from build123d import *

# Parameters (mm, degrees)
PAD015_DEPTH = 12
PAD014_DEPTH = 5


with BuildPart() as body013:
    # Sketch146 → Pad015 (new body)
    with BuildSketch(Plane.XY):
        with BuildLine():
            Line((41.956765, 0.26313), (41.959666, 5.256243))
            ThreePointArc((41.956765, 0.26313), (47.080742, 2.75671), (41.959666, 5.256243))
        make_face()
    extrude(amount=PAD015_DEPTH)


with BuildPart() as body013_1:
    # Body013 placement: moved
    add(body013.part.moved(Location((0, 0, 4))))


with BuildPart() as old_pinion:
    # Sketch145 → Pad014 (new body)
    with BuildSketch(Plane.XY):
        with BuildLine():
            Line((48.939875, 3.670275), (49.473913, 3.767638))
            Line((49.473913, 3.767638), (49.815259, 3.926647))
            Line((49.815259, 3.926647), (50.638101, 4.698494))
            ThreePointArc((50.638101, 4.698494), (50.5458, 4.994259), (50.440501, 5.285649))
            Line((50.440501, 5.285649), (49.318425, 5.40296))
            Line((49.318425, 5.40296), (48.950396, 5.323237))
            Line((48.950396, 5.323237), (48.466153, 5.077911))
            ThreePointArc((47.975725, 5.217399), (48.193585, 5.05148), (48.466153, 5.077911))
            ThreePointArc((47.975725, 5.217399), (47.866498, 5.389716), (47.749972, 5.557185))
            ThreePointArc((47.811432, 6.063346), (47.681442, 5.822318), (47.749972, 5.557185))
            Line((47.811432, 6.063346), (48.225241, 6.414684))
            Line((48.225241, 6.414684), (48.441351, 6.723062))
            Line((48.441351, 6.723062), (48.768029, 7.802923))
            ThreePointArc((48.768029, 7.802923), (48.540212, 8.012912), (48.303325, 8.212614))
            Line((48.303325, 8.212614), (47.272923, 7.75317))
            Line((47.272923, 7.75317), (46.994062, 7.500114))
            Line((46.994062, 7.500114), (46.697359, 7.045533))
            ThreePointArc((46.202892, 6.92112), (46.474523, 6.886359), (46.697359, 7.045533))
            ThreePointArc((46.202892, 6.92112), (46.022139, 7.015737), (45.837491, 7.102506))
            ThreePointArc((45.637635, 7.571584), (45.645575, 7.297853), (45.837491, 7.102506))
            Line((45.637635, 7.571584), (45.820336, 8.082756))
            Line((45.820336, 8.082756), (45.853303, 8.457875))
            Line((45.853303, 8.457875), (45.596285, 9.556401))
            ThreePointArc((45.596285, 9.556401), (45.293995, 9.624348), (44.988994, 9.678852))
            Line((44.988994, 9.678852), (44.326362, 8.765761))
            Line((44.326362, 8.765761), (44.211389, 8.407177))
            Line((44.211389, 8.407177), (44.181727, 7.865147))
            ThreePointArc((43.815712, 7.510168), (44.068332, 7.615881), (44.181727, 7.865147))
            ThreePointArc((43.815712, 7.510168), (43.611867, 7.501733), (43.408573, 7.484553))
            ThreePointArc((43.000954, 7.790859), (43.144695, 7.55777), (43.408573, 7.484553))
            Line((43.000954, 7.790859), (42.903591, 8.324897))
            Line((42.903591, 8.324897), (42.744582, 8.666243))
            Line((42.744582, 8.666243), (41.972735, 9.489085))
            ThreePointArc((41.972735, 9.489085), (41.67697, 9.396784), (41.38558, 9.291486))
            Line((41.38558, 9.291486), (41.268269, 8.169409))
            Line((41.268269, 8.169409), (41.347991, 7.80138))
            Line((41.347991, 7.80138), (41.593318, 7.317138))
            ThreePointArc((41.45383, 6.82671), (41.619749, 7.044569), (41.593318, 7.317138))
            ThreePointArc((41.45383, 6.82671), (41.281512, 6.717482), (41.114044, 6.600956))
            ThreePointArc((40.607883, 6.662416), (40.848911, 6.532426), (41.114044, 6.600956))
            Line((40.607883, 6.662416), (40.256545, 7.076225))
            Line((40.256545, 7.076225), (39.948167, 7.292335))
            Line((39.948167, 7.292335), (38.868306, 7.619013))
            ThreePointArc((38.868306, 7.619013), (38.658317, 7.391196), (38.458615, 7.154309))
            Line((38.458615, 7.154309), (38.918059, 6.123907))
            Line((38.918059, 6.123907), (39.171115, 5.845046))
            Line((39.171115, 5.845046), (39.625696, 5.548343))
            ThreePointArc((39.750109, 5.053876), (39.784869, 5.325508), (39.625696, 5.548343))
            ThreePointArc((39.750109, 5.053876), (39.655491, 4.873124), (39.568723, 4.688475))
            ThreePointArc((39.099644, 4.48862), (39.373376, 4.496559), (39.568723, 4.688475))
            Line((39.099644, 4.48862), (38.588472, 4.67132))
            Line((38.588472, 4.67132), (38.213354, 4.704288))
            Line((38.213354, 4.704288), (37.114828, 4.447269))
            ThreePointArc((37.114828, 4.447269), (37.046881, 4.144979), (36.992377, 3.839978))
            Line((36.992377, 3.839978), (37.905468, 3.177346))
            Line((37.905468, 3.177346), (38.264052, 3.062373))
            Line((38.264052, 3.062373), (38.806082, 3.032711))
            ThreePointArc((39.161061, 2.666696), (39.055348, 2.919317), (38.806082, 3.032711))
            ThreePointArc((39.161061, 2.666696), (39.169495, 2.462852), (39.186676, 2.259557))
            ThreePointArc((38.88037, 1.851938), (39.113458, 1.99568), (39.186676, 2.259557))
            Line((38.88037, 1.851938), (38.346331, 1.754575))
            Line((38.346331, 1.754575), (38.004985, 1.595567))
            Line((38.004985, 1.595567), (37.182144, 0.823719))
            ThreePointArc((37.182144, 0.823719), (37.274445, 0.527954), (37.379743, 0.236564))
            Line((37.379743, 0.236564), (38.50182, 0.119253))
            Line((38.50182, 0.119253), (38.869848, 0.198976))
            Line((38.869848, 0.198976), (39.354091, 0.444302))
            ThreePointArc((39.844519, 0.304814), (39.626659, 0.470733), (39.354091, 0.444302))
            ThreePointArc((39.844519, 0.304814), (39.953746, 0.132497), (40.070272, -0.034972))
            ThreePointArc((40.008813, -0.541133), (40.138803, -0.300105), (40.070272, -0.034972))
            Line((40.008813, -0.541133), (39.595004, -0.892471))
            Line((39.595004, -0.892471), (39.378894, -1.200849))
            Line((39.378894, -1.200849), (39.052216, -2.28071))
            ThreePointArc((39.052216, -2.28071), (39.280033, -2.490699), (39.516919, -2.690401))
            Line((39.516919, -2.690401), (40.547321, -2.230957))
            Line((40.547321, -2.230957), (40.826183, -1.977901))
            Line((40.826183, -1.977901), (41.122886, -1.52332))
            ThreePointArc((41.617353, -1.398907), (41.345721, -1.364146), (41.122886, -1.52332))
            ThreePointArc((41.617353, -1.398907), (41.798105, -1.493524), (41.982754, -1.580293))
            ThreePointArc((42.182609, -2.049371), (42.17467, -1.77564), (41.982754, -1.580293))
            Line((42.182609, -2.049371), (41.999908, -2.560543))
            Line((41.999908, -2.560543), (41.966941, -2.935662))
            Line((41.966941, -2.935662), (42.22396, -4.034188))
            ThreePointArc((42.22396, -4.034188), (42.52625, -4.102135), (42.831251, -4.156639))
            Line((42.831251, -4.156639), (43.493883, -3.243547))
            Line((43.493883, -3.243547), (43.608856, -2.884964))
            Line((43.608856, -2.884964), (43.638518, -2.342934))
            ThreePointArc((44.004532, -1.987955), (43.751912, -2.093668), (43.638518, -2.342934))
            ThreePointArc((44.004532, -1.987955), (44.208377, -1.97952), (44.411672, -1.96234))
            ThreePointArc((44.819291, -2.268646), (44.675549, -2.035557), (44.411672, -1.96234))
            Line((44.819291, -2.268646), (44.916653, -2.802684))
            Line((44.916653, -2.802684), (45.075662, -3.14403))
            Line((45.075662, -3.14403), (45.84751, -3.966872))
            ThreePointArc((45.84751, -3.966872), (46.143275, -3.874571), (46.434665, -3.769273))
            Line((46.434665, -3.769273), (46.551975, -2.647196))
            Line((46.551975, -2.647196), (46.472253, -2.279167))
            Line((46.472253, -2.279167), (46.226926, -1.794925))
            ThreePointArc((46.366415, -1.304496), (46.200495, -1.522356), (46.226926, -1.794925))
            ThreePointArc((46.366415, -1.304496), (46.538732, -1.195269), (46.7062, -1.078743))
            ThreePointArc((47.212362, -1.140203), (46.971333, -1.010213), (46.7062, -1.078743))
            Line((47.212362, -1.140203), (47.563699, -1.554012))
            Line((47.563699, -1.554012), (47.872078, -1.770122))
            Line((47.872078, -1.770122), (48.951939, -2.0968))
            ThreePointArc((48.951939, -2.0968), (49.161928, -1.868983), (49.36163, -1.632096))
            Line((49.36163, -1.632096), (48.902185, -0.601694))
            Line((48.902185, -0.601694), (48.649129, -0.322833))
            Line((48.649129, -0.322833), (48.194549, -0.02613))
            ThreePointArc((48.070135, 0.468337), (48.035375, 0.196706), (48.194549, -0.02613))
            ThreePointArc((48.070135, 0.468337), (48.164753, 0.649089), (48.251522, 0.833738))
            ThreePointArc((48.7206, 1.033593), (48.446869, 1.025654), (48.251522, 0.833738))
            Line((48.7206, 1.033593), (49.231772, 0.850893))
            Line((49.231772, 0.850893), (49.606891, 0.817925))
            Line((49.606891, 0.817925), (50.705417, 1.074944))
            ThreePointArc((50.705417, 1.074944), (50.773364, 1.377234), (50.827868, 1.682235))
            Line((50.827868, 1.682235), (49.914776, 2.344867))
            Line((49.914776, 2.344867), (49.556193, 2.45984))
            Line((49.556193, 2.45984), (49.014163, 2.489502))
            ThreePointArc((48.659184, 2.855517), (48.764896, 2.602897), (49.014163, 2.489502))
            ThreePointArc((48.659184, 2.855517), (48.650749, 3.059361), (48.633569, 3.262656))
            ThreePointArc((48.939875, 3.670275), (48.706786, 3.526534), (48.633569, 3.262656))
        make_face()
    extrude(amount=PAD014_DEPTH)


with BuildPart() as old_pinion_1:
    # Body012 placement: moved
    add(old_pinion.part.moved(Location((0, 0, 4))))

    # Cut001: cut Body013
    add(body013_1.part, mode=Mode.SUBTRACT)


with BuildPart() as old_pinion_2:
    # Cut001 placement: moved
    add(old_pinion_1.part.moved(Location((0, 0, 25.5))))


solid = old_pinion_2.part
Read the model definition and answer for the solid it produces. Units are mm, in the model's axes. A direction names the side the tool comes from. Round coordinates to 2 decimals unless told otherwise and drop trailing zeros. Use one line per item in the form item = value. Start each with the question number.
(1) Flat-ended cylindrical pins translate along their axes: pin 1 Ø1.5 at (x, z) = (39, 30.5) entering from -Y; pin 2 Ø8 at (x, y) = (46.5, 3.5) entering from -Z; pin 3 Ø1 at (y, z) = (7, 33.5) entering from +X; pin 4 Ø1 at (y, z) = (8, 33.5) entering from +X. Find the tip coordinate at first contact, or state that the pin passes through.
(2) For faces 1 (the face through (44.662, 9.229, 31.965)), 2 (the face through (43.158, -3.706, 31.965)), 3 (the face through (38.685, 6.646, 31.965)), determine the directions among +Z, -Z, +X, -X, +Y, -Y from which every point of the face is accessible in a straight line to the end or side of a thin tool.
(3) Determine the mould class of faces 4 (the face through (37.93, 0.18, 31.96)), 5 (the face through (48.602, 7.255, 31.965)), 6 (the face through (49.887, 5.343, 31.965)) for opening direction Y: +Y half, -Y half, draft (parallel to the pull), parting line (faces both ways), or undercut.
(4) Find the intervals of material crossed by line 1 along Y through (x, z) = (38.75, 31.1); line 2 along Y through (x, z) = (50, 30.7); line 3 along Y through (x, z) = (47.75, 33.7), in increasing order. Write a range as from..to.
Checked values:
q1.pin_1 = -2.69
q1.pin_2 = 29.5
q1.pin_3 = 48.68
q1.pin_4 = 48.77
q2.face_1 = +Z, -Z, +Y
q2.face_2 = +Z, -Z, -Y
q2.face_3 = +Z, -Z, -X
q3.face_4 = -Y half
q3.face_5 = undercut
q3.face_6 = +Y half
q4.line_1 = 0.17..1.83, 3.04..4.61, 6.5..7.49
q4.line_2 = 0.91..2.28, 4.1..5.33
q4.line_3 = -1.68..5.56, 6..7.97
